For this review, take the finished solid that the model builds, in its own axes (mm). Face numbers are marked on the shaded views. A direction names the side the tool comes from. Give positions to 0.01 mm unless a question says otherwise; leave off trailing zeros. Write each loop counter-clockwise with the first axis right and the second up, starting at its lowest first coordinate (ties: lowest second). Pieces come first, ordered by that corner, then holes. Notation, with made-up numbers: M 67,45 L 114,45 A15 ccw 114,58 Z; hole C 32.25,82.25 d6. An arc over 180 degrees is marked long. Answer as a JSON object with one key per item and string values. Group by question number.
```python
from build123d import *

# Parameters (mm, degrees)
SKETCH_1_W          = 40
SKETCH_1_H          = 40
EXTRUDE_1_DEPTH     = 100
CUT_EXTRUDE_1_REACH = 131.283
SKETCH_2_R          = 3.5
SKETCH_2_R_2        = 3
FILLET_1_R          = 5
SKETCH_3_R          = 1.236693346
CUT_EXTRUDE_2_DEPTH = 0.5


with BuildPart() as part:
    # 草图1 → 凸台-拉伸1 (new body)
    with BuildSketch(Plane(origin=(0, 0, 0), x_dir=(0, 0, -1), z_dir=(1, 0, 0))):
        with Locations((40.704960836, 35.035758607)):
            Rectangle(SKETCH_1_W, SKETCH_1_H)
    extrude(amount=EXTRUDE_1_DEPTH)

    # 草图2 → 切除-拉伸1 (cut, up to next)
    with BuildSketch(Plane(origin=(100, 0, 0), x_dir=(0, 0, -1), z_dir=(1, 0, 0)), mode=Mode.PRIVATE) as cut_extrude_1_sk1:
        with Locations((40.704960836, 35.035758607)):
            Circle(SKETCH_2_R)
    cut_extrude_1_tool1 = extrude(cut_extrude_1_sk1.sketch, amount=-CUT_EXTRUDE_1_REACH, mode=Mode.PRIVATE) & part.part
    # 草图2 → 切除-拉伸1 (cut, up to next)
    with BuildSketch(Plane(origin=(100, 0, 0), x_dir=(0, 0, -1), z_dir=(1, 0, 0)), mode=Mode.PRIVATE) as cut_extrude_1_sk2:
        with Locations((25.854960836, 49.885758607)):
            Circle(SKETCH_2_R_2)
    cut_extrude_1_tool2 = extrude(cut_extrude_1_sk2.sketch, amount=-CUT_EXTRUDE_1_REACH, mode=Mode.PRIVATE) & part.part
    # 草图2 → 切除-拉伸1 (cut, up to next)
    with BuildSketch(Plane(origin=(100, 0, 0), x_dir=(0, 0, -1), z_dir=(1, 0, 0)), mode=Mode.PRIVATE) as cut_extrude_1_sk3:
        with Locations((25.854960836, 20.185758607)):
            Circle(SKETCH_2_R_2)
    cut_extrude_1_tool3 = extrude(cut_extrude_1_sk3.sketch, amount=-CUT_EXTRUDE_1_REACH, mode=Mode.PRIVATE) & part.part
    # 草图2 → 切除-拉伸1 (cut, up to next)
    with BuildSketch(Plane(origin=(100, 0, 0), x_dir=(0, 0, -1), z_dir=(1, 0, 0)), mode=Mode.PRIVATE) as cut_extrude_1_sk4:
        with Locations((55.554960836, 49.885758607)):
            Circle(SKETCH_2_R_2)
    cut_extrude_1_tool4 = extrude(cut_extrude_1_sk4.sketch, amount=-CUT_EXTRUDE_1_REACH, mode=Mode.PRIVATE) & part.part
    # 草图2 → 切除-拉伸1 (cut, up to next)
    with BuildSketch(Plane(origin=(100, 0, 0), x_dir=(0, 0, -1), z_dir=(1, 0, 0)), mode=Mode.PRIVATE) as cut_extrude_1_sk5:
        with Locations((55.554960836, 20.185758607)):
            Circle(SKETCH_2_R_2)
    cut_extrude_1_tool5 = extrude(cut_extrude_1_sk5.sketch, amount=-CUT_EXTRUDE_1_REACH, mode=Mode.PRIVATE) & part.part
    # 草图2 → 切除-拉伸1 (cut, up to next)
    with BuildSketch(Plane(origin=(100, 0, 0), x_dir=(0, 0, -1), z_dir=(1, 0, 0)), mode=Mode.PRIVATE) as cut_extrude_1_sk6:
        Polygon((36.704960836, 15.035758607), (36.704960836, 19.535758607), (34.004960836, 19.535758607), (34.004960836, 17.735758607), (31.004960836, 17.735758607), (31.004960836, 22.235758607), (35.704960836, 27.275758607), (45.704960836, 27.275758607), (50.404960836, 22.235758607), (50.404960836, 17.735758607), (47.404960836, 17.735758607), (47.404960836, 19.535758607), (44.704960836, 19.535758607), (44.704960836, 15.035758607), align=None)
    cut_extrude_1_tool6 = extrude(cut_extrude_1_sk6.sketch, amount=-CUT_EXTRUDE_1_REACH, mode=Mode.PRIVATE) & part.part
    # 草图2 → 切除-拉伸1 (cut, up to next)
    with BuildSketch(Plane(origin=(100, 0, 0), x_dir=(0, 0, -1), z_dir=(1, 0, 0)), mode=Mode.PRIVATE) as cut_extrude_1_sk7:
        Polygon((44.704960836, 55.035758607), (44.704960836, 50.535758607), (47.404960836, 50.535758607), (47.404960836, 52.335758607), (50.404960836, 52.335758607), (50.404960836, 47.835758607), (45.704960836, 42.795758607), (35.704960836, 42.795758607), (31.004960836, 47.835758607), (31.004960836, 52.335758607), (34.004960836, 52.335758607), (34.004960836, 50.535758607), (36.704960836, 50.535758607), (36.704960836, 55.035758607), align=None)
    cut_extrude_1_tool7 = extrude(cut_extrude_1_sk7.sketch, amount=-CUT_EXTRUDE_1_REACH, mode=Mode.PRIVATE) & part.part
    # 草图2 → 切除-拉伸1 (cut, up to next)
    with BuildSketch(Plane(origin=(100, 0, 0), x_dir=(0, 0, -1), z_dir=(1, 0, 0)), mode=Mode.PRIVATE) as cut_extrude_1_sk8:
        Polygon((20.704960836, 31.035758607), (20.704960836, 39.035758607), (25.204960836, 39.035758607), (25.204960836, 41.735758607), (23.404960836, 41.735758607), (23.404960836, 44.735758607), (27.954960836, 44.735758607), (32.944960836, 40.035758607), (32.944960836, 30.035758607), (27.954960836, 25.335758607), (23.404960836, 25.335758607), (23.404960836, 28.335758607), (25.204960836, 28.335758607), (25.204960836, 31.035758607), align=None)
    cut_extrude_1_tool8 = extrude(cut_extrude_1_sk8.sketch, amount=-CUT_EXTRUDE_1_REACH, mode=Mode.PRIVATE) & part.part
    # 草图2 → 切除-拉伸1 (cut, up to next)
    with BuildSketch(Plane(origin=(100, 0, 0), x_dir=(0, 0, -1), z_dir=(1, 0, 0)), mode=Mode.PRIVATE) as cut_extrude_1_sk9:
        Polygon((60.704960836, 31.035758607), (56.204960836, 31.035758607), (56.204960836, 28.335758607), (58.004960836, 28.335758607), (58.004960836, 25.335758607), (53.454960836, 25.335758607), (48.464960836, 30.035758607), (48.464960836, 40.035758607), (53.454960836, 44.735758607), (58.004960836, 44.735758607), (58.004960836, 41.735758607), (56.204960836, 41.735758607), (56.204960836, 39.035758607), (60.704960836, 39.035758607), align=None)
    cut_extrude_1_tool9 = extrude(cut_extrude_1_sk9.sketch, amount=-CUT_EXTRUDE_1_REACH, mode=Mode.PRIVATE) & part.part
    add(cut_extrude_1_tool1.solids().sort_by_distance((100, 35.035759, -40.704961))[0], mode=Mode.SUBTRACT)
    add(cut_extrude_1_tool2.solids().sort_by_distance((100, 49.885759, -25.854961))[0], mode=Mode.SUBTRACT)
    add(cut_extrude_1_tool3.solids().sort_by_distance((100, 20.185759, -25.854961))[0], mode=Mode.SUBTRACT)
    add(cut_extrude_1_tool4.solids().sort_by_distance((100, 49.885759, -55.554961))[0], mode=Mode.SUBTRACT)
    add(cut_extrude_1_tool5.solids().sort_by_distance((100, 20.185759, -55.554961))[0], mode=Mode.SUBTRACT)
    add(cut_extrude_1_tool6.solids().sort_by_distance((100, 21.537481, -40.704961))[0], mode=Mode.SUBTRACT)
    add(cut_extrude_1_tool7.solids().sort_by_distance((100, 48.534036, -40.704961))[0], mode=Mode.SUBTRACT)
    add(cut_extrude_1_tool8.solids().sort_by_distance((100, 35.035759, -27.209927))[0], mode=Mode.SUBTRACT)
    add(cut_extrude_1_tool9.solids().sort_by_distance((100, 35.035759, -54.199995))[0], mode=Mode.SUBTRACT)

    # 圆角1
    fillet_1_edges = [part.edges().sort_by_distance(p)[0] for p in [
        (50, 55.035758607, -20.704960836),
        (50, 55.035758607, -60.704960836),
        (50, 15.035758607, -60.704960836),
        (50, 15.035758607, -20.704960836),
    ]]
    fillet(fillet_1_edges, radius=FILLET_1_R)

    # 草图3 → 切除-拉伸2 (cut)
    with BuildSketch(Plane(origin=(0, 42.795758607, 0), x_dir=(1, 0, 0), z_dir=(0, 1, 0))):
        with Locations(Location((50, 40.704960836, 0), (0, 0, 270))):
            Circle(SKETCH_3_R)
    extrude(amount=-CUT_EXTRUDE_2_DEPTH, mode=Mode.SUBTRACT)


solid = part.part
```
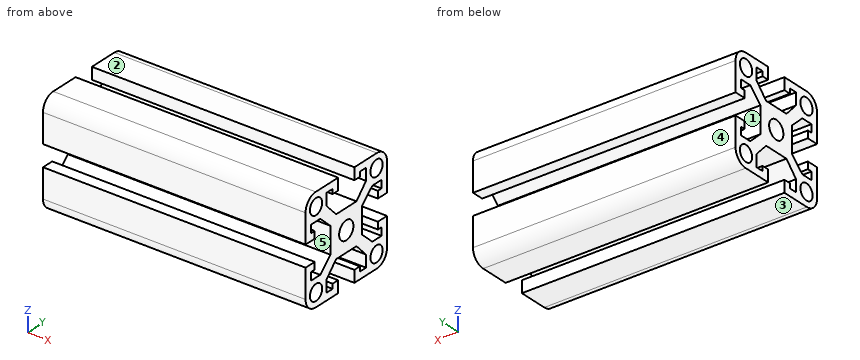
Item 1: To check wall thickness, follow probe 1 along Z at (x, y) = (63, 31); probe 2 along Y at (x, z) = (25.5, -36); probe 3 along Y at (x, z) = (14, -26). State the ranges of each line that lie inside material, in increasing order.
Item 2: Consider section D-D (x = 56.5). State how many separate pieces and enclosed holes the cut face has, plus the area to 3 significant figures.
Item 3: Consider section C-C (z = -40.5). Give the boundary of the cut face in (x, y).
Item 4: Consider section B-B (y = 36.5). Give the boundary of the cut face in (x, z).
Item 5: Consider section A-A (z = -51.5). Give the boundary of the cut face in (x, y), plus the area to 3 significant figures.
Item 6: Insertion check: P1, Ø0.5, axis at x = 36, z = -56.5, coming from the +Y side; P2, Ø4, axis at x = 74, z = -42.5, coming from the +Y side; P3, Ø4, axis at x = 54, y = 33.5, coming from the -Z side. Each pin has a flat end and moves straight along its axis. Give the tip position at first contact, or say it passes through.
Item 7: Machinability: for the marked faces 4 and 5, which of the approach directions +Z, -Z, +X, -X, +Y, -Y give a long, thin tool a straight path to every point of the face, cutting with its end or side? Answer none if there is none.
Item 8: Draft analysis for pull direction Z (two halves, no side actions). For the marked faces 1, 2 and 3, state which applies: released by +Z, released by -Z, zero draft, split by the parting line, or undercut.
Result set:
{
 "1": {"probe 1": "z = -60.7 to -56.2, -48.46 to -32.94, -25.2 to -20.7", "probe 2": "y = 15.04 to 19.54, 27.28 to 42.8, 50.54 to 55.04", "probe 3": "y = 15.04 to 17.19, 23.18 to 25.34, 44.74 to 46.89, 52.88 to 55.04"},
 "2": {"separate pieces": "1", "enclosed holes": "5", "area": "733 mm^2"},
 "3": {"outline": "M 0,27.28 L 100,27.28 L 100,31.54 L 0,31.54 Z; M 0,38.53 L 100,38.53 L 100,42.8 L 51.22,42.8 L 51.22,42.3 L 48.78,42.3 L 48.78,42.8 L 0,42.8 Z"},
 "4": {"outline": "M 0,-48.46 L 100,-48.46 L 100,-43.88 L 0,-43.88 Z; M 0,-37.53 L 100,-37.53 L 100,-32.94 L 0,-32.94 Z"},
 "5": {"outline": "M 0,15.04 L 100,15.04 L 100,27.18 L 0,27.18 Z; M 0,42.89 L 100,42.89 L 100,55.04 L 0,55.04 Z", "area": "2,430 mm^2"},
 "6": {"P1": "stops at y = 55.01", "P2": "stops at y = 42.8", "P3": "stops at z = -48.46"},
 "7": {"face 4": "+Z, -Z, +X, -X, +Y", "face 5": "+X, -X"},
 "8": {"face 1": "undercut", "face 2": "released by +Z", "face 3": "released by -Z"}
}
